from build123d import *

# Parameters (mm, degrees)
F1_DEPTH  = 19
F2_R      = 24
F3_DEPTH  = 25
F4_R      = 9.99999
F5_R      = 5
F6_DEPTH  = 25
F7_R      = 7.5
F8_DEPTH  = 10
F9_W      = 6
F9_H      = 19
F10_DEPTH = 25
F11_DEPTH = 25
F12_R     = 4.25
F13_DEPTH = 250
F15_DEPTH = 8
F16_R     = 4.25
F17_DEPTH = 250
F18_R     = 9.49999


# Not quite as in the source:
# - a fillet or chamfer is up to 0.001 mm smaller than in the source, because OpenCascade refuses the exact size


with BuildPart() as f1:
    # F0 (on Top) → F1 (new body)
    with BuildSketch(Plane.XY):
        Polygon((0, 90), (-40, 90), (-40, 70), (-70, 70), (-70, 40), (-90, 40), (-90, 0), (0, 0), align=None)
        Polygon((40, 90), (0, 90), (0, 0), (90, 0), (90, 40), (70, 40), (70, 70), (40, 70), align=None)
        Polygon((0, -90), (0, 0), (-90, 0), (-90, -40), (-70, -40), (-70, -70), (-40, -70), (-40, -90), align=None)
        Polygon((90, 0), (0, 0), (0, -90), (40, -90), (40, -70), (70, -70), (70, -40), (90, -40), align=None)
    extrude(amount=F1_DEPTH)

    # F2 (on face) → F3 (cut)
    with BuildSketch(Plane.XY.offset(19)):
        Circle(F2_R)
    extrude(amount=-F3_DEPTH, mode=Mode.SUBTRACT)

    # F4 (radius 10 in the source; OpenCascade refuses exactly that, so slightly less here)
    f4_edges = [f1.edges().sort_by_distance(p)[0] for p in [
        (-70, 40, 9.5),
        (-40, 70, 9.5),
        (-40, 90, 9.5),
        (-70, 70, 9.5),
        (-90, 40, 9.5),
        (-40, -90, 9.5),
        (-40, -70, 9.5),
        (-70, -70, 9.5),
        (-70, -40, 9.5),
        (-90, -40, 9.5),
        (40, -90, 9.5),
        (40, -70, 9.5),
        (70, -70, 9.5),
        (70, -40, 9.5),
        (90, -40, 9.5),
        (90, 40, 9.5),
        (70, 40, 9.5),
        (70, 70, 9.5),
        (40, 70, 9.5),
        (40, 90, 9.5),
    ]]
    fillet(f4_edges, radius=F4_R)

    # F5 (on face) → F6 (cut)
    with BuildSketch(Plane.XY.offset(19)):
        with Locations((-50, -50)):
            Circle(F5_R)
        with Locations((50, -50)):
            Circle(F5_R)
        with Locations((-50, 50)):
            Circle(F5_R)
        with Locations((50, 50)):
            Circle(F5_R)
    extrude(amount=-F6_DEPTH, mode=Mode.SUBTRACT)

    # F7 (on face) → F8 (cut)
    with BuildSketch(Plane(origin=(0, 0, 0), x_dir=(1, 0, 0), z_dir=(0, 0, -1))):
        with Locations((-50, 50)):
            Circle(F7_R)
        with Locations((50, 50)):
            Circle(F7_R)
        with Locations((-50, -50)):
            Circle(F7_R)
        with Locations((50, -50)):
            Circle(F7_R)
    extrude(amount=-F8_DEPTH, mode=Mode.SUBTRACT)

    # F9 (on face) → F10 (join)
    with BuildSketch(Plane.YZ.offset(90)):
        with Locations((-27, 9.5)):
            Rectangle(F9_W, F9_H)
        with Locations((27, 9.5)):
            Rectangle(F9_W, F9_H)
    extrude(amount=F10_DEPTH)

    # F9 (on face) → F11 (join)
    with BuildSketch(Plane.YZ.offset(90)):
        with Locations((-27, 9.5)):
            Rectangle(F9_W, F9_H)
        with Locations((27, 9.5)):
            Rectangle(F9_W, F9_H)
    extrude(amount=F11_DEPTH)

    # F12 (on face) → F13 (cut)
    with BuildSketch(Plane.XZ.offset(30)):
        with BuildLine():
            ThreePointArc((125, 0), (134.5, 9.5), (125, 19))
            Line((125, 19), (115, 19))
            Line((115, 19), (115, 0))
            Line((115, 0), (125, 0))
        make_face()
        with Locations((125, 9.5)):
            Circle(F12_R, mode=Mode.SUBTRACT)
        with Locations((125, 9.5)):
            Circle(F12_R)
    extrude(amount=-F13_DEPTH, mode=Mode.SUBTRACT)

    # F15 (add): faces of the model
    f15_faces = [f1.faces().sort_by_distance(p)[0] for p in [
        (115, -27, 9.5),
        (115, 27, 9.5),
    ]]
    extrude(f15_faces, amount=F15_DEPTH)

    # F16 (on face) → F17 (cut)
    with BuildSketch(Plane.XZ.offset(30)):
        with Locations((115.5, 9.5)):
            Circle(F16_R)
    extrude(amount=-F17_DEPTH, mode=Mode.SUBTRACT)

    # F18 (radius 9.5 in the source; OpenCascade refuses exactly that, so slightly less here)
    f18_edges = [f1.edges().sort_by_distance(p)[0] for p in [
        (123, 27, 0),
        (123, -27, 0),
        (123, -27, 19),
        (123, 27, 19),
    ]]
    fillet(f18_edges, radius=F18_R)


solid = f1.part
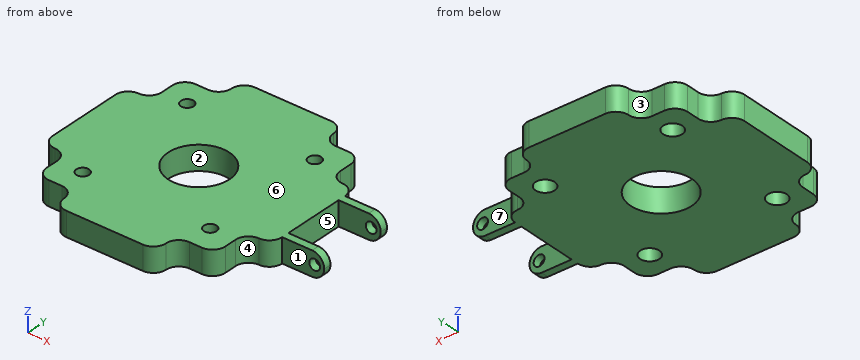
Work out the finished part from the listing and answer in its coordinate system (mm). Face numbers are marked on the shaded views. A direction names the side the tool comes from. Give positions to 0.01 mm unless a question says otherwise; leave off trailing zeros. Loops run counter-clockwise (first coordinate to the right, second up) from the corner with the lowest first, then second, coordinate; pieces in that order, holes last. Notation, with made-up numbers: (-1.5, 5) -> (57.5, 5) arc R17 ccw to (57.5, 33) -> close; hole circle Ø9 at (65.25, 33.5). An arc over 180 degrees is marked (long way). Use a Markdown table: item, result. Add a question column.
1. Section D-D on y = 62.5 is taken. Determine the outline of the cut face in (x, z).
2. For the marked faces 5, 6 and 7, determine the directions among +Z, -Z, +X, -X, +Y, -Y from which every point of the face is accessible in a straight line to the end or side of a thin tool.
3. Section B-B on x = 101.5 is taken. Determine the outline of the cut face in (y, z), and give its area (3 significant figures).
4. Section A-A on y = 0 is taken. Determine the outline of the cut face in (x, z), and give its area (3 significant figures).
5. Find the intervals of material crossed by probe 1 along Y at (x, z) = (50, 4); probe 2 along Y at (x, z) = (50, 16.5); probe 3 along Y at (x, z) = (96, 1.5), in increasing order.
6. Determine the mould class of the marked faces 1, 2, 3 and 4 for opening direction X: released by +X, released by -X, zero draft, split by the parting line, or undercut.
7. Flat-ended cylindrical pins translate along their axes: pin 1 Ø11 at (x, z) = (-52.5, 10.5) entering from +Y; pin 2 Ø9.5 at (x, z) = (104.5, 7) entering from +Y; pin 3 Ø4 at (x, y) = (51, -58.5) entering from -Z; pin 4 Ø5 at (x, z) = (115.5, 9.5) entering from +Y. Find the tip coordinate at first contact, or state that the pin passes through.
Results below:
| question | item | result |
|---|---|---|
| 1 | outline | (-69.68, 0) -> (69.68, 0) -> (69.68, 19) -> (-69.68, 19) -> close |
| 2 | face 5 | +Z, -Z, +X |
| 2 | face 6 | +Z, +X, -X, +Y, -Y |
| 2 | face 7 | +Z, -Z, +X, +Y |
| 3 | outline | (-30, 0) -> (-24, 0) -> (-24, 19) -> (-30, 19) -> close; (24, 0) -> (30, 0) -> (30, 19) -> (24, 19) -> close |
| 3 | area | 228 mm^2 |
| 4 | outline | (-90, 0) -> (-24, 0) -> (-24, 19) -> (-90, 19) -> close; (24, 0) -> (90, 0) -> (90, 19) -> (24, 19) -> close |
| 4 | area | 2,510 mm^2 |
| 5 | probe 1 | y = -70 to -57.5, -42.5 to 42.5, 57.5 to 70 |
| 5 | probe 2 | y = -70 to -55, -45 to 45, 55 to 70 |
| 5 | probe 3 | y = -30 to -24, 24 to 30 |
| 6 | face 1 | zero draft |
| 6 | face 2 | undercut |
| 6 | face 3 | released by -X |
| 6 | face 4 | released by +X |
| 7 | pin 1 | stops at y = 70.46 |
| 7 | pin 2 | stops at y = 30 |
| 7 | pin 3 | stops at z = 0 |
| 7 | pin 4 | passes through |
